Answer from the drawing. Dimensions are ordinates in mm from the lowest x, y and z of the part. A direction names the side the tool comes from. Give positions to 0.01 mm unless a question says otherwise; leave off trailing zeros. Write each loop counter-clockwise with the first axis right and the second up, starting at its lowest first coordinate (ties: lowest second). Pieces come first, ordered by that corner, then holes.
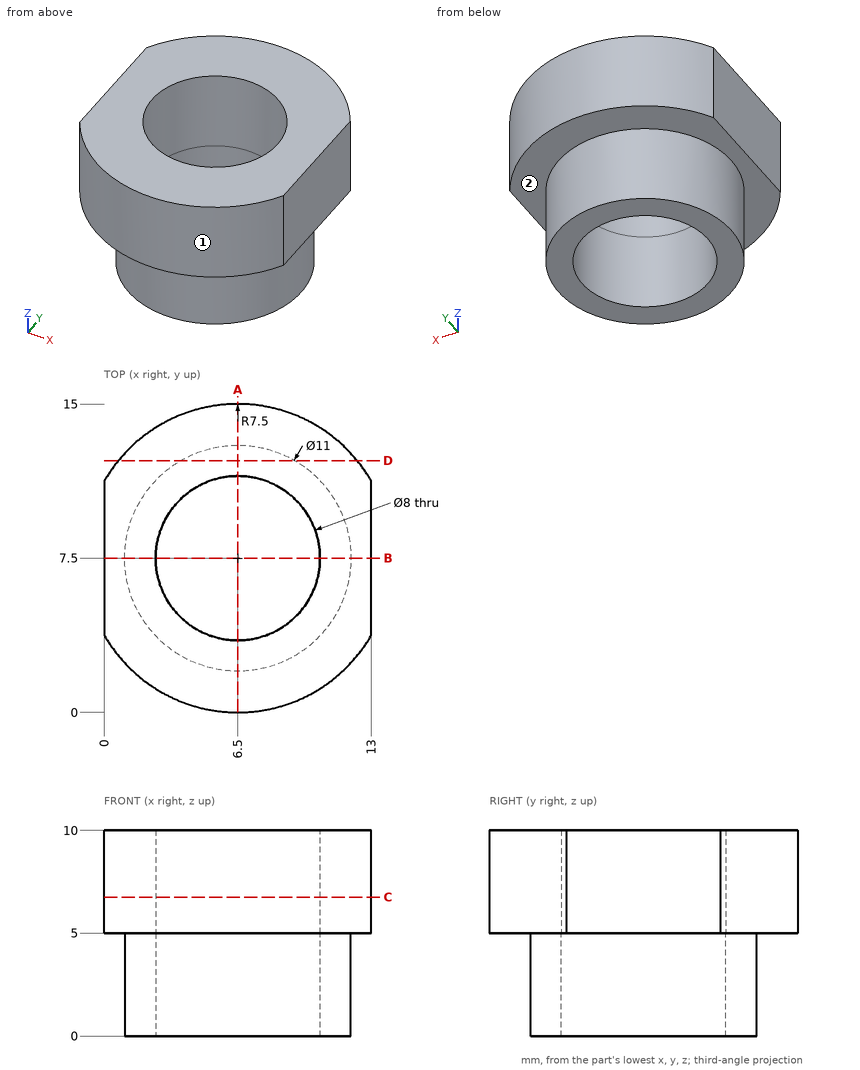
Item 1: This flat-tipped pin is pushed along its axis until it touches: pin 1 Ø1 at (x, y) = (8, 7.5) entering from -Z. Where does it stop, or does it pass through?
Result set:
pin 1: passes through
Item 2: Section D-D (y = 12.25) is taken. Write down the section's boundary in (x, z), and give its area (3 significant figures).
Result set:
outline: (0.7, 5) - (3.73, 5) - (3.73, 0) - (9.27, 0) - (9.27, 5) - (12.3, 5) - (12.3, 10) - (0.7, 10) - close
area: 85.8 mm2
Item 3: Find the intervals of material crossed by line 1 along X through (y, z) = (7.5, 6.9); line 2 along Y through (x, z) = (6.5, 1.65); line 3 along Y through (x, z) = (10, 7.5), in increasing order.
Result set:
line 1: x = 0 to 2.5, 10.5 to 13
line 2: y = 2 to 3.5, 11.5 to 13
line 3: y = 0.87 to 5.56, 9.44 to 14.13
Item 4: Section C-C (z = 6.75) is taken. Write down the section's boundary in (x, y), and give its area (3 significant figures).
Result set:
outline: (0, 3.76) arc R7.5 ccw to (13, 3.76) - (13, 11.24) arc R7.5 ccw to (0, 11.24) - close; hole circle Ø8 at (6.5, 7.5)
area: 116 mm2
Item 5: Section B-B (y = 7.5) is taken. Write down the section's boundary in (x, z), and give its area (3 significant figures).
Result set:
outline: (0, 5) - (1, 5) - (1, 0) - (2.5, 0) - (2.5, 10) - (0, 10) - close; (10.5, 0) - (12, 0) - (12, 5) - (13, 5) - (13, 10) - (10.5, 10) - close
area: 40.0 mm2
Item 6: Which of the six approach directions +Z, -Z, +X, -X, +Y, -Y give full straight-line access (tool end or side, diameter ignored) to the marked faces 1 and 2?
Result set:
face 1: +Z, -Z, -Y
face 2: -Z
Item 7: Section A-A (x = 6.5) is taken. Write down the section's boundary in (y, z), and give its area (3 significant figures).
Result set:
outline: (0, 5) - (2, 5) - (2, 0) - (3.5, 0) - (3.5, 10) - (0, 10) - close; (11.5, 0) - (13, 0) - (13, 5) - (15, 5) - (15, 10) - (11.5, 10) - close
area: 50.0 mm2
